Model file for the job. Use its own axes, mm. Face numbers are marked on the shaded views. A direction names the side the tool comes from. Coordinates: 2 decimals unless noted, no trailing zeros. Order: outer loops, then holes, each group sorted by start corner. A loop starts at its lowest first (then second) coordinate and runs counter-clockwise, first axis right, second up. Notation, with made-up numbers: (20, 82.25) -> (65, 82.25) arc R25 ccw to (65, 109.25) -> close; hole circle Ø2 at (85, -12). An arc over 180 degrees is marked (long way). Return JSON: item names as keys, results as strings. Group by question number.
1) Cut at A-A (x = 8). Write the cut outline in (y, z), and give its area (4 significant figures).
2) Flat gauge pins, fed straight in: pin 1 (0.8 mm diameter, centred on y = 8.5, z = -1.5, fed in from +X); pin 2 (1.2 mm diameter, centred on x = 10, z = -1, fed in from -Y); pin 3 (2 mm diameter, centred on x = 18, y = 10, fed in from -Z). Where does each tip first touch, or does it go through?
3) Cut at D-D (x = 23.75). Write the cut outline in (y, z), and give its area (3 significant figures).
4) Which spindle directions (+Z, -Z, +X, -X, +Y, -Y) get a long thin tool onto all of the face, cutting with end or side? Do the marked faces 4 and 5. Say none if no direction does.
5) Pull direction X, two halves, no side cores. Call the marked faces 1, 2 and 3: +X half, -X half, draft (parallel to the pull), parting line (faces both ways), or undercut.
6) Cut at C-C (y = 10.25). Write the cut outline in (x, z), and give its area (3 significant figures).
7) Probe line 1 (Y direction, x = 8, z = -1.5); line 2 (Y direction, x = 8, z = 0.8); line 3 (Z direction, x = 20, y = 12.5). List the from-to ranges inside material, lowest first.
from build123d import *

# Parameters (mm, degrees)
SKETCH_1_W          = 25
SKETCH_1_H          = 13
EXTRUDE_1_DEPTH     = 1.5
SKETCH_2_R          = 2
CUT_EXTRUDE_1_DEPTH = 2.8
SKETCH_3_W          = 15
SKETCH_3_H          = 11
EXTRUDE_2_DEPTH     = 2.5
FILLET_1_R          = 5.5
CHAMFER_1_SIZE      = 1


with BuildPart() as part:
    # 草图1 → 凸台-拉伸1 (new body)
    with BuildSketch(Plane.XY):
        with Locations((12.5, 6.5)):
            Rectangle(SKETCH_1_W, SKETCH_1_H)
    extrude(amount=EXTRUDE_1_DEPTH)

    # 草图2 → 切除-拉伸1 (cut)
    with BuildSketch(Plane.XY.offset(1.5)):
        with Locations((8, 6.5)):
            Circle(SKETCH_2_R)
    extrude(amount=-CUT_EXTRUDE_1_DEPTH, mode=Mode.SUBTRACT)

    # 草图3 → 凸台-拉伸2 (add)
    with BuildSketch(Plane(origin=(0, 0, 0), x_dir=(-1, 0, 0), z_dir=(0, 0, -1))):
        with Locations((-8.976194502, 6.5)):
            Rectangle(SKETCH_3_W, SKETCH_3_H)
        with BuildLine():
            Line((-7.25, 8.08113883), (-7.200635773, 4.943235139))
            ThreePointArc((-7.200635773, 4.943235139), (-9.749783493, 6.472473116), (-7.25, 8.08113883))
        make_face(mode=Mode.SUBTRACT)
    extrude(amount=EXTRUDE_2_DEPTH)

    # 圆角1
    fillet_1_edges = [part.edges().sort_by_distance(p)[0] for p in [
        (1.476194502, 1, -1.25),
        (1.476194502, 12, -1.25),
    ]]
    fillet(fillet_1_edges, radius=FILLET_1_R - 0.0001)  # a hair under: the kernel refuses the full size

    # 倒角1
    chamfer_1_edges = [part.edges().sort_by_distance(p)[0] for p in [
        (16.476194502, 12, -1.25),
        (16.476194502, 1, -1.25),
    ]]
    chamfer(chamfer_1_edges, length=CHAMFER_1_SIZE)


solid = part.part
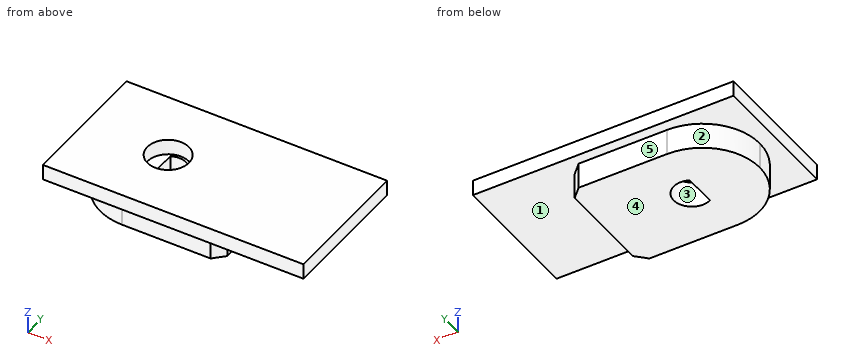
Answers below:
{
 "1": {"outline": "(0, 0) -> (1, 0) -> (1, -2.5) -> (4.75, -2.5) -> (4.75, 0) -> (4.5, 0) -> (4.5, 1.5) -> (0, 1.5) -> close; (8.25, -2.5) -> (12, -2.5) -> (12, 0) -> (13, 0) -> (13, 1.5) -> (8.5, 1.5) -> (8.5, 0) -> (8.25, 0) -> close", "area": "32.25 mm^2"},
 "2": {"pin 1": "stops at x = 16.48", "pin 2": "stops at y = 1", "pin 3": "stops at z = 0"},
 "3": {"outline": "(0, 0) -> (13, 0) -> (13, 1.5) -> (0, 1.5) -> close", "area": "19.5 mm^2"},
 "4": {"face 4": "-Z, +X, -X, +Y, -Y", "face 5": "-Z, +X, -X, +Y"},
 "5": {"face 1": "draft", "face 2": "-X half", "face 3": "undercut"},
 "6": {"outline": "(0, 0) -> (2.95, 0) -> (2.95, -2.5) -> (16.48, -2.5) -> (16.48, 0) -> (25, 0) -> (25, 1.5) -> (0, 1.5) -> close", "area": "71.3 mm^2"},
 "7": {"line 1": "y = 1 to 4.75, 8.25 to 12", "line 2": "y = 0 to 4.5, 8.5 to 13", "line 3": "z = 0 to 1.5"}
}
